from build123d import *

# Parameters (mm, degrees)
SKETCH1_R            = 40
SKETCH1_R_2          = 25
BOSS_EXTRUDE1_DEPTH  = 2
M5_CLEARANCE_HOLE1_D = 5.3
CIRPATTERN1_COUNT    = 12


with BuildPart() as part:
    # Sketch1 → Boss-Extrude1 (new body)
    with BuildSketch(Plane.XY):
        Circle(SKETCH1_R)
        Circle(SKETCH1_R_2, mode=Mode.SUBTRACT)
    extrude(amount=BOSS_EXTRUDE1_DEPTH)

    # M5 Clearance Hole1 (through all)
    with Locations(Plane.XY.offset(2)):
        with Locations((0, 32.5)):
            m5_clearance_hole1 = Hole(M5_CLEARANCE_HOLE1_D / 2)

    # CirPattern1: M5 Clearance Hole1 ×12 about axis
    cirpattern1_axis = Axis((0, 0, 0), (0, 0, 1))
    for i in range(1, CIRPATTERN1_COUNT):
        add(m5_clearance_hole1.rotate(cirpattern1_axis, i * 360 / CIRPATTERN1_COUNT), mode=Mode.SUBTRACT)


solid = part.part
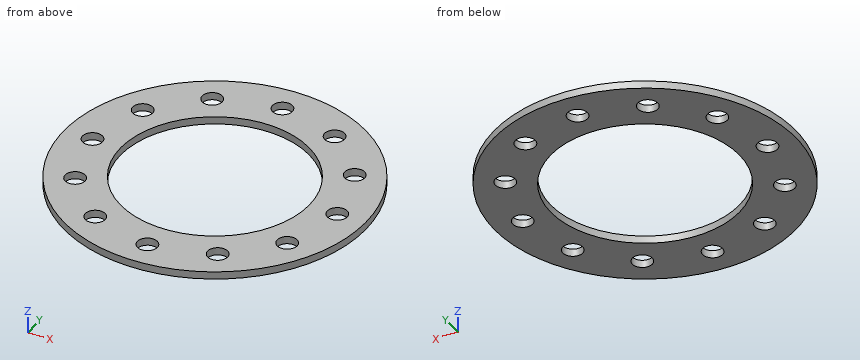
Geometry check sheet. Reference: the model listing, model coordinates, mm. Give positions to 0.01 mm unless a question says otherwise; leave off trailing zeros. Write each loop counter-clockwise with the first axis right and the second up, starting at its lowest first coordinate (ties: lowest second). Pieces come first, ordered by that corner, then holes.
1) Cross-section at C-C (x = -28). Record the boundary of the cut face in (y, z).
Values follow:
outline: (-28.57, 0) - (-18.9, 0) - (-18.9, 2) - (-28.57, 2) - close; (-13.6, 0) - (13.6, 0) - (13.6, 2) - (-13.6, 2) - close; (18.9, 0) - (28.57, 0) - (28.57, 2) - (18.9, 2) - close
2) Thickness scan on line 1 (X direction, y = -1.5, z = 1.25); line 2 (Y direction, x = 1, z = 1.1); line 3 (Y direction, x = -8, z = 1.95). Record the ranges inside material, lowest first.
Values follow:
line 1: x = -39.97 to -34.68, -30.32 to -24.95, 24.95 to 30.32, 34.68 to 39.97
line 2: y = -39.99 to -34.95, -30.05 to -24.98, 24.98 to 30.05, 34.95 to 39.99
line 3: y = -39.19 to -23.69, 23.69 to 39.19
3) Cross-section at A-A (x = 0). Record the boundary of the cut face in (y, z).
Values follow:
outline: (-40, 0) - (-35.15, 0) - (-35.15, 2) - (-40, 2) - close; (-29.85, 0) - (-25, 0) - (-25, 2) - (-29.85, 2) - close; (25, 0) - (29.85, 0) - (29.85, 2) - (25, 2) - close; (35.15, 0) - (40, 0) - (40, 2) - (35.15, 2) - close
4) Cross-section at D-D (z = 1.5). Count the separate pieces of the cut face and the enclosed holes in it, plus the area to 3 significant figures.
Values follow:
separate pieces: 1
enclosed holes: 13
area: 2,800 mm2
